Check sheet for the modelled part. Datum: model origin and axes. Units: mm. Face numbers are marked on the shaded views. A direction names the side the tool comes from. Give positions to 0.01 mm unless a question says otherwise; leave off trailing zeros. Loops run counter-clockwise (first coordinate to the right, second up) from the corner with the lowest first, then second, coordinate; pieces in that order, holes last. Notation, with made-up numbers: (84.25, 62) -> (122.25, 62) arc R13 cw to (122.25, 76) -> close; hole circle Ø11 at (34.25, 51.25). An arc over 180 degrees is marked (long way). Write each question's results on one line, items separated by ' | '. Start each with the question number.
1. Cross-section at B-B on y = 19. Record the boundary of the cut face in (x, z), and give its area (3 significant figures).
2. Cross-section at C-C on x = -21.5. Record the boundary of the cut face in (y, z), and give its area (3 significant figures).
3. Cross-section at A-A on y = 0. Record the boundary of the cut face in (x, z), and give its area (3 significant figures).
4. Material ranges on L1, parallel to X at y = 19, z = 1.15; L2, parallel to Y at x = 0, z = 1.25; L3, parallel to Y at x = -21.5, z = 0.6, recorded low to high. Write a range as from..to.
5. Cross-section at D-D on x = -10. Record the boundary of the cut face in (y, z), and give its area (3 significant figures).
6. Tool access check on the marked faces 1, 2 and 3. Record the directions out of +Z, -Z, +X, -X, +Y, -Y that give a thin tool (end or side, any length) a straight path to the whole face; none if there is none.
7. Gauge pin test, flat ends, axial feed: pin 1 Ø5 at (y, z) = (11, 3.5) entering from -X; pin 2 Ø8 at (x, y) = (-6.5, -23.5) entering from +Z. Record the tip position at first contact, or that the pin passes through.
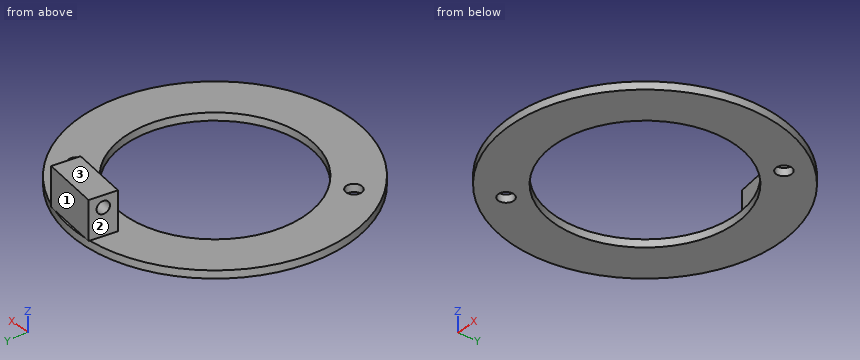
from build123d import *

# Parameters (mm, degrees)
F0_R     = 35
F0_R_2   = 23.5
F1_DEPTH = 2
F2_R     = 2
F3_DEPTH = 2.001
F5_DEPTH = 10
F6_R     = 1.6
F7_DEPTH = 46.636965


with BuildPart() as f1:
    # F0 (on Top) → F1 (new body)
    with BuildSketch(Plane.XY):
        Circle(F0_R)
        Circle(F0_R_2, mode=Mode.SUBTRACT)
    extrude(amount=F1_DEPTH)

    # F2 (on Top) → F3 (cut, through all)
    with BuildSketch(Plane.XY):
        with Locations((-21.5, -19)):
            Circle(F2_R)
        with Locations((21.5, 19)):
            Circle(F2_R)
    extrude(amount=F3_DEPTH, mode=Mode.SUBTRACT)

    # F4 (on face) → F5 (join)
    with BuildSketch(Plane.XY.offset(2)):
        Polygon((11.80901, 33.238829), (-2.764145, 35.165779), (-3.68174, 28.226181), (10.891415, 26.299231), align=None)
    extrude(amount=F5_DEPTH)

    # F6 (on face) → F7 (cut, through all)
    with BuildSketch(Plane(origin=(-7.286578, 0.963475, 0), x_dir=(-0.131085, -0.991371, 0), z_dir=(-0.991371, 0.131085, 0))):
        with Locations((-31, 9)):
            Circle(F6_R)
    extrude(amount=-F7_DEPTH, mode=Mode.SUBTRACT)


solid = f1.part
Geometry says:
1) outline: (-29.39, 0) -> (-13.83, 0) -> (-13.83, 2) -> (-29.39, 2) -> close; (13.83, 0) -> (19.5, 0) -> (19.5, 2) -> (13.83, 2) -> close; (23.5, 0) -> (29.39, 0) -> (29.39, 2) -> (23.5, 2) -> close | area: 54.3 mm^2
2) outline: (-27.62, 0) -> (-21, 0) -> (-21, 2) -> (-27.62, 2) -> close; (-17, 0) -> (-9.49, 0) -> (-9.49, 2) -> (-17, 2) -> close; (9.49, 0) -> (27.62, 0) -> (27.62, 2) -> (9.49, 2) -> close | area: 64.5 mm^2
3) outline: (-35, 0) -> (-23.5, 0) -> (-23.5, 2) -> (-35, 2) -> close; (23.5, 0) -> (35, 0) -> (35, 2) -> (23.5, 2) -> close | area: 46.0 mm^2
4) L1: -29.39..-13.83, 13.83..19.5, 23.5..29.39 | L2: -35..-23.5, 23.5..35 | L3: -27.62..-21, -17..-9.49, 9.49..27.62
5) outline: (-33.54, 0) -> (-21.27, 0) -> (-21.27, 2) -> (-33.54, 2) -> close; (21.27, 0) -> (33.54, 0) -> (33.54, 2) -> (21.27, 2) -> close | area: 49.1 mm^2
6) face 1: +Z, +X, +Y | face 2: +Z, -X, +Y | face 3: +Z, +X, -X, +Y, -Y
7) pin 1: x = -33.82 | pin 2: z = 2
